Geometry: final body of the model. Coordinates: model frame, mm. A direction names the side the tool comes from. Coordinates: 2 decimals unless noted, no trailing zeros. Write each loop counter-clockwise with the first axis right and the second up, starting at its lowest first coordinate (ties: lowest second). Pieces come first, ordered by that corner, then holes. Notation, with made-up numbers: (-15, 15) -> (2, 15) arc R20 cw to (2, 45) -> close; hole circle Ø8 at (-7, 21). An arc over 180 degrees is marked (long way). Answer as a JSON object with one key per item and string values. Group by question number.
```python
from build123d import *

# Parameters (mm, degrees)
SKETCH1_W           = 60
SKETCH1_H           = 75
BOSS_EXTRUDE1_DEPTH = 12
SKETCH6_W           = 8.75
SKETCH6_H           = 8
BOSS_EXTRUDE2_DEPTH = 9
SKETCH3_R           = 2.65
SKETCH3_R_2         = 11
CUT_EXTRUDE4_DEPTH  = 53.414215629
SKETCH5_R           = 20
SKETCH5_R_2         = 2.65
SKETCH5_R_3         = 11
CUT_EXTRUDE8_DEPTH  = 5
DOVE_CUT_DEPTH      = 58.447802395
DOVE_CUT_DEPTH_BACK = 58.447802395
BOSS_EXTRUDE3_DEPTH = 10
CHAMFER1_SIZE       = 15
SKETCH16_R          = 1.75
CUT_EXTRUDE9_DEPTH  = 105.880884817


with BuildPart() as part:
    # Sketch1 → Boss-Extrude1 (new body)
    with BuildSketch(Plane(origin=(0, 0, 0), x_dir=(1, 0, 0), z_dir=(0, 1, 0))):
        Rectangle(SKETCH1_W, SKETCH1_H)
    extrude(amount=BOSS_EXTRUDE1_DEPTH)

    # Sketch6 → Boss-Extrude2 (add)
    with BuildSketch(Plane.XZ):
        with Locations((-5.625, -24)):
            Rectangle(SKETCH6_W, SKETCH6_H)
        with Locations((5.625, -24)):
            Rectangle(SKETCH6_W, SKETCH6_H)
        with Locations((5.625, 24)):
            Rectangle(SKETCH6_W, SKETCH6_H)
        with Locations((-5.625, 24)):
            Rectangle(SKETCH6_W, SKETCH6_H)
    extrude(amount=BOSS_EXTRUDE2_DEPTH)

    # Sketch3 → Cut-Extrude4 (cut, through all)
    with BuildSketch(Plane(origin=(0, 12, 0), x_dir=(1, 0, 0), z_dir=(0, 1, 0))):
        with Locations(Location((-5, 24, 0), (0, 0, 270))):
            Circle(SKETCH3_R)
        with Locations(Location((5, 24, 0), (0, 0, 90))):
            Circle(SKETCH3_R)
        with Locations(Location((5, -24, 0), (0, 0, 270))):
            Circle(SKETCH3_R)
        with Locations(Location((-5, -24, 0), (0, 0, 90))):
            Circle(SKETCH3_R)
        with Locations(Location((0, -10, 0), (0, 0, 270))):
            Circle(SKETCH3_R_2)
    extrude(amount=-CUT_EXTRUDE4_DEPTH, mode=Mode.SUBTRACT)

    # Sketch5 → Cut-Extrude8 (cut)
    with BuildSketch(Plane(origin=(0, 12, 0), x_dir=(1, 0, 0), z_dir=(0, 1, 0))):
        with Locations(Location((0, -10, 0), (0, 0, 270))):
            Circle(SKETCH5_R)
        with Locations(Location((-5, -24, 0), (0, 0, 270))):
            Circle(SKETCH5_R_2, mode=Mode.SUBTRACT)
        with Locations(Location((0, -10, 0), (0, 0, 270))):
            Circle(SKETCH5_R_3, mode=Mode.SUBTRACT)
        with Locations(Location((5, -24, 0), (0, 0, 270))):
            Circle(SKETCH5_R_2, mode=Mode.SUBTRACT)
    extrude(amount=-CUT_EXTRUDE8_DEPTH, mode=Mode.SUBTRACT)

    # Sketch15 → Dove Cut (cut, two sides: drawn at the far end of the back side and taken through both)
    with BuildSketch(Plane(origin=(0, 0, 10), x_dir=(0, 0, 1), z_dir=(-1, 0, 0)).offset(-DOVE_CUT_DEPTH_BACK)):
        Polygon((-21.91084373, 6.75), (-12, 6.75), (-12, 12), (-20, 12), (-22.41084373, 6.75), align=None)
        Polygon((12, 12), (20, 12), (22.41084373, 6.75), (21.91084373, 6.75), (12, 6.75), align=None)
    extrude(amount=DOVE_CUT_DEPTH + DOVE_CUT_DEPTH_BACK, mode=Mode.SUBTRACT)

    # Sketch8 → Boss-Extrude3 (add)
    with BuildSketch(Plane(origin=(-30, 30, 0), x_dir=(0, 1, 0), z_dir=(1, 0, 0))):
        Polygon((-30, 37.5), (-50, 37.5), (-50, -90), (-30, -90), (-18, -90), (-18, -37.5), (-30, -37.5), align=None)
    extrude(amount=BOSS_EXTRUDE3_DEPTH)

    # Chamfer1
    chamfer1_edges = [part.edges().sort_by_distance(p)[0] for p in [
        (-20, 6, -37.5),
    ]]
    chamfer(chamfer1_edges, length=CHAMFER1_SIZE)

    # Sketch16 → Cut-Extrude9 (cut, through all)
    with BuildSketch(Plane(origin=(-20, 0, 0), x_dir=(0, 0, -1), z_dir=(1, 0, 0))):
        with Locations((77.5, -12.5)):
            Circle(SKETCH16_R)
        with Locations((32.5, -12.5)):
            Circle(SKETCH16_R)
    extrude(amount=-CUT_EXTRUDE9_DEPTH, mode=Mode.SUBTRACT)


solid = part.part
```
Item 1: Contact query for flat-ended pins moving along their axis: pin 1 (1.5 mm diameter, centred on x = 9.5, y = -7, fed in from +Z); pin 2 (1.5 mm diameter, centred on x = 0, z = -7, fed in from -Y); pin 3 (6.5 mm diameter, centred on x = 3.5, z = 25.5, fed in from -Y). Output: stop coordinate, or through.
Item 2: Section B-B on x = 0. Output: boundary loops of the cut face in (y, z).
Item 3: Mould query, pull axis Z, two halves, no side actions, for faces 1 (the flat face through (20, 9, -2)), 2 (the flat face through (-10, -4, 24)), 3 (the flat face through (12, 6, -37.5)). Classes: +Z half, -Z half, draft (parallel to the pull), parting line (faces both ways), or undercut.
Item 4: Section C-C on x = 26. Output: boundary loops of the cut face in (y, z).
Item 5: Section D-D on z = -32.5. Output: boundary loops of the cut face in (x, y).
Item 6: Section A-A on z = 24. Output: boundary loops of the cut face in (x, y), then the cut area to 3 significant figures.
Item 7: Ray query, L1, parallel to X at y = -3, z = 24; L2, parallel to X at y = 2, z = 24; L3, parallel to Y at x = -25.25, z = -77.5. Return the intervals inside material, ascending. Write a range as [from, to].
Item 8: Set-up query: faces 4 (the flat face through (8, -9, 25)), 5 (the flat face through (-4.2, 7, 20.5)), 6 (the flat face through (-1.25, -4, 24)), 7 (the flat face through (0, 6.75, -7)). Return all of +Z, -Z, +X, -X, +Y, -Y with unobstructed straight access to the full face (end or side cutting, diameter ignored); none if empty.
Answer sheet:
{
 "1": {"pin 1": "stops at z = 28", "pin 2": "stops at y = 0", "pin 3": "stops at y = -9"},
 "2": {"outline": "(0, -37.5) -> (12, -37.5) -> (12, -10) -> (6.75, -12.41) -> (6.75, -2) -> (7, -2) -> (7, -1) -> (0, -1) -> close; (0, 21) -> (7, 21) -> (7, 22) -> (6.75, 22) -> (6.75, 32.41) -> (12, 30) -> (12, 37.5) -> (0, 37.5) -> close"},
 "3": {"face 1": "undercut", "face 2": "draft", "face 3": "-Z half"},
 "4": {"outline": "(0, -37.5) -> (12, -37.5) -> (12, -10) -> (6.75, -12.41) -> (6.75, -2) -> (12, -2) -> (12, 22) -> (6.75, 22) -> (6.75, 32.41) -> (12, 30) -> (12, 37.5) -> (0, 37.5) -> close"},
 "5": {"outline": "(-30, -20) -> (-20, -20) -> (-20, -14.25) -> (-30, -14.25) -> close; (-30, -10.75) -> (-20, -10.75) -> (-20, 0) -> (30, 0) -> (30, 12) -> (-30, 12) -> close"},
 "6": {"outline": "(-30, -20) -> (-20, -20) -> (-20, 0) -> (-10, 0) -> (-10, -9) -> (-7.65, -9) -> (-7.65, 6.75) -> (-30, 6.75) -> close; (-2.35, -9) -> (-1.25, -9) -> (-1.25, 0) -> (1.25, 0) -> (1.25, -9) -> (2.35, -9) -> (2.35, 6.75) -> (-2.35, 6.75) -> close; (7.65, -9) -> (10, -9) -> (10, 0) -> (30, 0) -> (30, 6.75) -> (7.65, 6.75) -> close", "area": "596 mm^2"},
 "7": {"L1": "x = [-30, -20], [-10, -7.65], [-2.35, -1.25], [1.25, 2.35], [7.65, 10]", "L2": "x = [-30, -7.65], [-2.35, 2.35], [7.65, 30]", "L3": "y = [-20, -14.25], [-10.75, 12]"},
 "8": {"face 4": "+Z, -Z, +X, -Y", "face 5": "+Y", "face 6": "+Z, -Z, -Y", "face 7": "+X, -X"}
}
